```python
from build123d import *

# Parameters (mm, degrees)
SKETCH_1_R          = 1.525
EXTRUDE_1_DEPTH     = 1.5
SKETCH_2_R          = 1.525
CUT_EXTRUDE_1_DEPTH = 21
CUT_EXTRUDE_2_DEPTH = 11
CUT_EXTRUDE_3_DEPTH = 11
FILLET_1_R          = 8
SKETCH_5_W          = 69
SKETCH_5_H          = 49
CUT_EXTRUDE_4_DEPTH = 11
FILLET_2_R          = 2
FILLET_3_R          = 2


with BuildPart() as part:
    # 草图1 → 凸台-拉伸1 (new, symmetric)
    with BuildSketch(Plane.XY):
        Polygon((-70.5, -18), (-70.5, 18), (-55.5, 35), (55.5, 35), (70.5, 18), (70.5, -18), (55.5, -35), (-55.5, -35), align=None)
        with Locations((67.5, -15)):
            Circle(SKETCH_1_R, mode=Mode.SUBTRACT)
        with Locations((-67.5, -15)):
            Circle(SKETCH_1_R, mode=Mode.SUBTRACT)
        with Locations((-67.5, 15)):
            Circle(SKETCH_1_R, mode=Mode.SUBTRACT)
        with Locations((67.5, 15)):
            Circle(SKETCH_1_R, mode=Mode.SUBTRACT)
    extrude(amount=EXTRUDE_1_DEPTH, both=True)

    # 草图2 → 切除-拉伸1 (cut, symmetric)
    with BuildSketch(Plane(origin=(0, 0, -1.5), x_dir=(-1, 0, 0), z_dir=(0, 0, -1))):
        with Locations((-24, 21)):
            Circle(SKETCH_2_R)
        with Locations((-24, -21)):
            Circle(SKETCH_2_R)
        with Locations((51, 21)):
            Circle(SKETCH_2_R)
        with Locations((51, -21)):
            Circle(SKETCH_2_R)
    extrude(amount=CUT_EXTRUDE_1_DEPTH, both=True, mode=Mode.SUBTRACT)

    # 草图3 → 切除-拉伸2 (cut, symmetric)
    with BuildSketch(Plane(origin=(0, 0, -1.5), x_dir=(-1, 0, 0), z_dir=(0, 0, -1))):
        Polygon((-70.5, 18), (-60.5, 18), (-45.5, 35), (-55.5, 35), align=None)
        Polygon((55.5, 35), (70.5, 18), (60.5, 18), (45.5, 35), align=None)
    extrude(amount=CUT_EXTRUDE_2_DEPTH, both=True, mode=Mode.SUBTRACT)

    # 草图4 → 切除-拉伸3 (cut, symmetric)
    with BuildSketch(Plane(origin=(0, 0, -1.5), x_dir=(-1, 0, 0), z_dir=(0, 0, -1))):
        Polygon((-55.205882353, 24), (55.205882353, 24), (45.5, 35), (-45.5, 35), align=None)
    extrude(amount=CUT_EXTRUDE_3_DEPTH, both=True, mode=Mode.SUBTRACT)

    # 圆角1
    fillet_1_edges = [part.edges().sort_by_distance(p)[0] for p in [
        (55.205882353, 24, 0),
        (-55.205882353, 24, 0),
        (60.5, 18, 0),
        (-60.5, 18, 0),
    ]]
    fillet(fillet_1_edges, radius=FILLET_1_R)

    # 草图5 → 切除-拉伸4 (cut, symmetric)
    with BuildSketch(Plane(origin=(0, 0, -1.5), x_dir=(-1, 0, 0), z_dir=(0, 0, -1))):
        with Locations((13.5, -5.5)):
            Rectangle(SKETCH_5_W, SKETCH_5_H)
        Polygon((-55.5, 15.140970914), (-27, 19.072005396), (-27, -30), (-49.242791484, -30), (-55.5, -22.908497015), align=None)
    extrude(amount=CUT_EXTRUDE_4_DEPTH, both=True, mode=Mode.SUBTRACT)

    # 圆角2
    fillet_2_edges = [part.edges().sort_by_distance(p)[0] for p in [
        (-48, 19, 0),
        (-48, -30, 0),
        (21, -30, 0),
        (21, 19, 0),
        (55.5, -22.908497015, 0),
        (55.5, 15.140970914, 0),
        (27, 19.072005396, 0),
        (27, -30, 0),
        (49.242791484, -30, 0),
    ]]
    fillet(fillet_2_edges, radius=FILLET_2_R)

    # 圆角3
    fillet_3_edges = [part.edges().sort_by_distance(p)[0] for p in [
        (70.5, 18, 0),
        (70.5, -18, 0),
        (55.5, -35, 0),
        (-55.5, -35, 0),
        (-70.5, -18, 0),
        (-70.5, 18, 0),
    ]]
    fillet(fillet_3_edges, radius=FILLET_3_R)


solid = part.part
```
Check sheet for the modelled part. Datum: model origin and axes. Units: mm. A direction names the side the tool comes from. Coordinates: 2 decimals unless noted, no trailing zeros. Loops run counter-clockwise (first coordinate to the right, second up) from the corner with the lowest first, then second, coordinate; pieces in that order, holes last.
1) Release check for a two-part mould opening along X. For faces 4 (the face through (-66.1, 14.4, 0)), 5 (the face through (-62.951, -26.555, 0.021)), 6 (the face through (54.93, 23.27, 0.02)) record: released by +X, released by -X, zero draft, split by the parting line, or undercut.
2) Sectioned sample at B-B (y = -15). Record the boundary of the cut face in (x, z) (3 decimals), and give its area (3 significant figures).
3) Sectioned sample at D-D (y = 3.5). Record the boundary of the cut face in (x, z).
4) Gauge pin test, flat ends, axial feed: pin 1 (4 mm diameter, centred on x = 24, y = -21, fed in from +Z); pin 2 (0.9 mm diameter, centred on x = 67, z = 0.5, fed in from +Y). Record the tip position at first contact, or that the pin passes through.
5) Sectioned sample at A-A (x = -43.5). Record the boundary of the cut face in (y, z), and give its area (3 significant figures).
6) Sectioned sample at C-C (x = 24). Record the boundary of the cut face in (y, z) (3 decimals), and give its area (3 significant figures).
7) Access from +Z, -Z, +X, -X, +Y, -Y to the whole of each face (thin tool, end or side, straight path). Record for faces 1 (the face through (55.5, -5, 0)), 2 (the face through (-66, 18, 0)), 3 (the face through (-70.5, -1, 0)).
8) Material ranges on probe 1 along Y at (x, z) = (24, 0.7) (3 decimals); probe 2 along X at (y, z) = (-2, -1); probe 3 along Y at (x, z) = (0, 1.25), recorded low to high.
Check sheet entries:
1. face 4: undercut
1. face 5: released by -X
1. face 6: released by +X
2. outline: (-70.5, -1.5) - (-69.025, -1.5) - (-69.025, 1.5) - (-70.5, 1.5) - close; (-65.975, -1.5) - (-48, -1.5) - (-48, 1.5) - (-65.975, 1.5) - close; (21, -1.5) - (27, -1.5) - (27, 1.5) - (21, 1.5) - close; (55.5, -1.5) - (65.975, -1.5) - (65.975, 1.5) - (55.5, 1.5) - close; (69.025, -1.5) - (70.5, -1.5) - (70.5, 1.5) - (69.025, 1.5) - close
2. area: 112 mm2
3. outline: (-70.5, -1.5) - (-48, -1.5) - (-48, 1.5) - (-70.5, 1.5) - close; (21, -1.5) - (27, -1.5) - (27, 1.5) - (21, 1.5) - close; (55.5, -1.5) - (70.5, -1.5) - (70.5, 1.5) - (55.5, 1.5) - close
4. pin 1: stops at z = 1.5
4. pin 2: stops at y = 18
5. outline: (-35, -1.5) - (-30, -1.5) - (-30, 1.5) - (-35, 1.5) - close; (19, -1.5) - (24, -1.5) - (24, 1.5) - (19, 1.5) - close
5. area: 30.0 mm2
6. outline: (-35, -1.5) - (-22.525, -1.5) - (-22.525, 1.5) - (-35, 1.5) - close; (-19.475, -1.5) - (19.475, -1.5) - (19.475, 1.5) - (-19.475, 1.5) - close; (22.525, -1.5) - (24, -1.5) - (24, 1.5) - (22.525, 1.5) - close
6. area: 159 mm2
7. face 1: +Z, -Z
7. face 2: +Z, -Z, -X, +Y
7. face 3: +Z, -Z, -X, +Y, -Y
8. probe 1: y = -35 to -22.525, -19.475 to 19.475, 22.525 to 24
8. probe 2: x = -70.5 to -48, 21 to 27, 55.5 to 70.5
8. probe 3: y = -35 to -30, 19 to 24
